Model file for the job. Use its own axes, mm. Face numbers are marked on the shaded views. Coordinates: 2 decimals unless noted, no trailing zeros. Write each loop counter-clockwise with the first axis right and the second up, starting at its lowest first coordinate (ties: lowest second). Pieces come first, ordered by that corner, then holes. Notation, with made-up numbers: (57.5, -19) -> (89.5, -19) arc R16 cw to (89.5, -7) -> close; hole circle Ø4 at (20, 35.5). An arc over 180 degrees is marked (long way). Answer as a JSON object with one key per item and string values. Group by question number.
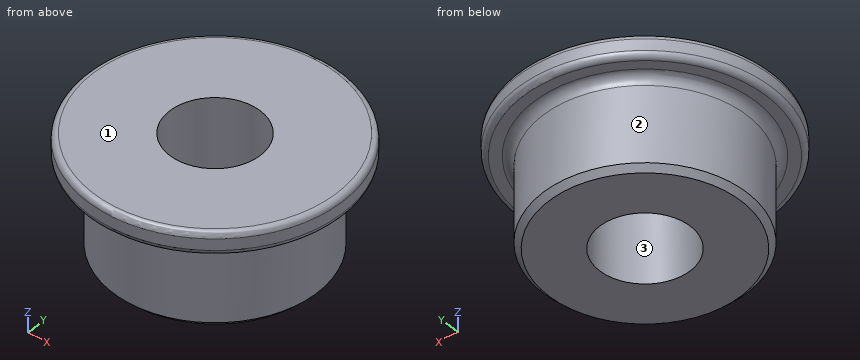
from build123d import *

# Parameters (mm, degrees)
SKETCH1_R           = 9
SKETCH1_R_2         = 4
BOSS_EXTRUDE1_DEPTH = 8
BOSS_EXTRUDE2_START = 2
SKETCH2_R           = 11.25
SKETCH2_R_2         = 4
BOSS_EXTRUDE2_DEPTH = 2
FILLET1_R           = 0.5
FILLET2_R           = 0.5
FILLET3_R           = 0.8
CHAMFER1_SIZE       = 0.5


with BuildPart() as part:
    # Sketch1 → Boss-Extrude1 (new body)
    with BuildSketch(Plane.XY):
        Circle(SKETCH1_R)
        Circle(SKETCH1_R_2, mode=Mode.SUBTRACT)
    extrude(amount=-BOSS_EXTRUDE1_DEPTH)

    # Sketch2 → Boss-Extrude2 (add)
    with BuildSketch(Plane.XY.offset(BOSS_EXTRUDE2_START)):
        Circle(SKETCH2_R)
        Circle(SKETCH2_R_2, mode=Mode.SUBTRACT)
    extrude(amount=-BOSS_EXTRUDE2_DEPTH)

    # Fillet1
    fillet1_edges = [part.edges().sort_by_distance(p)[0] for p in [
        (-11.25, 0, 2),
    ]]
    fillet(fillet1_edges, radius=FILLET1_R)

    # Fillet2
    fillet2_edges = [part.edges().sort_by_distance(p)[0] for p in [
        (-11.25, 0, 0),
    ]]
    fillet(fillet2_edges, radius=FILLET2_R)

    # Fillet3
    fillet3_edges = [part.edges().sort_by_distance(p)[0] for p in [
        (-9, 0, 0),
    ]]
    fillet(fillet3_edges, radius=FILLET3_R)

    # Chamfer1
    chamfer1_edges = [part.edges().sort_by_distance(p)[0] for p in [
        (-9, 0, -8),
    ]]
    chamfer(chamfer1_edges, length=CHAMFER1_SIZE)


solid = part.part
(1) Cut at A-A on x = 0. List the corners of the cut face in (y, z).
(2) Cut at C-C on z = -4.25. List the corners of the cut face in (x, y).
(3) Pull direction Y, two halves, no side cores. Call the marked faces 1, 2 and 3: released by +Y, released by -Y, zero draft, split by the parting line, or undercut.
(4) Pin check, flat tips, straight feed: pin 1 (2 mm diameter, centred on y = 2, z = -1.5, fed in from +X); pin 2 (4 mm diameter, centred on y = 1.5, z = -3.5, fed in from -X); pin 3 (3 mm diameter, centred on x = -3, z = -5, fed in from +Y). Stop position of each tip, or through.
(5) Wall check: probe 1 along Y at (x, z) = (0, -4.5); probe 2 along X at (y, z) = (-2, -3); probe 3 along X at (y, z) = (0.25, -3). Give the ranges that are in metal, low to high.
Results found:
{
 "1": {"outline": "(-11.25, 0.5) arc R0.5 ccw to (-10.75, 0) -> (-9.8, 0) arc R0.8 cw to (-9, -0.8) -> (-9, -7.5) -> (-8.5, -8) -> (-4, -8) -> (-4, 2) -> (-10.75, 2) arc R0.5 ccw to (-11.25, 1.5) -> close; (4, -8) -> (8.5, -8) -> (9, -7.5) -> (9, -0.8) arc R0.8 cw to (9.8, 0) -> (10.75, 0) arc R0.5 ccw to (11.25, 0.5) -> (11.25, 1.5) arc R0.5 ccw to (10.75, 2) -> (4, 2) -> close"},
 "2": {"outline": "circle Ø18 at (0, 0); hole circle Ø8 at (0, 0)"},
 "3": {"face 1": "zero draft", "face 2": "split by the parting line", "face 3": "undercut"},
 "4": {"pin 1": "stops at x = 8.94", "pin 2": "stops at x = -9", "pin 3": "stops at y = 8.87"},
 "5": {"probe 1": "y = -9 to -4, 4 to 9", "probe 2": "x = -8.77 to -3.46, 3.46 to 8.77", "probe 3": "x = -9 to -3.99, 3.99 to 9"}
}
